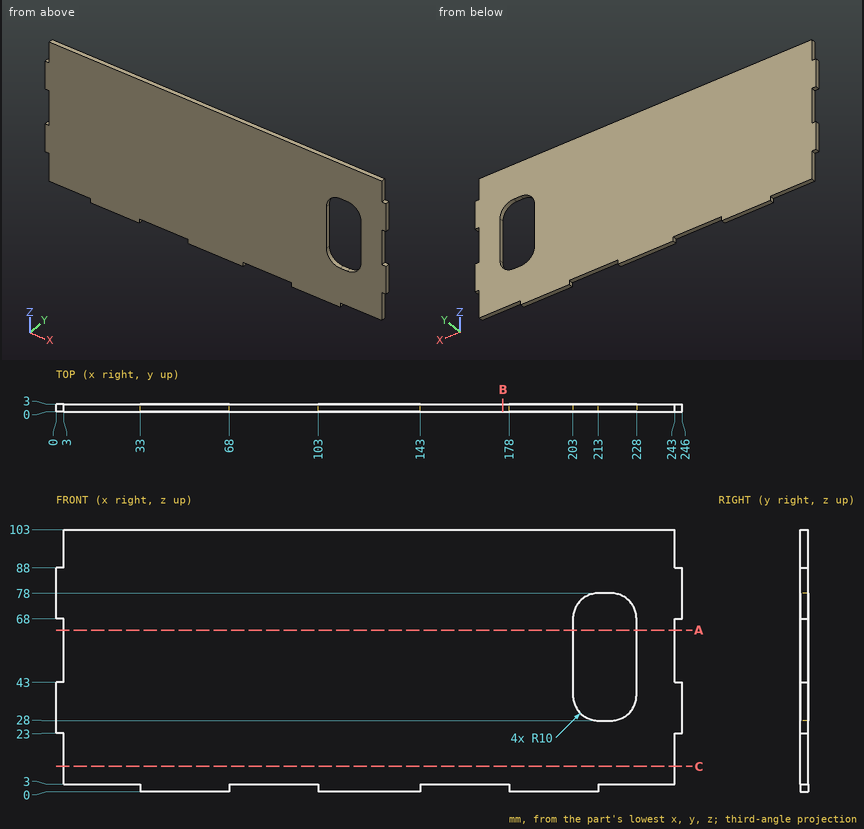
For this review, use the dimensioned drawing (mm, ordinates from the lowest corner) and the shaded views. Give positions to 0.01 mm unless a question says otherwise; leave off trailing zeros. Write each loop counter-clockwise with the first axis right and the second up, starting at its lowest first coordinate (ties: lowest second). Pieces come first, ordered by that corner, then holes. Notation, with made-up numbers: M 68,66 L 89,66 A11 cw 89,86 Z; hole C 77,71 d10. An arc over 180 degrees is marked long. Answer as a JSON object with one key per item and string values. Group by question number.
Item 1: For pin 1 Ø0.9 at (x, y) = (244.5, 2) entering from +Z; pin 2 Ø0.9 at (y, z) = (1, 1) entering from -X; pin 3 Ø1.5 at (x, y) = (17, 1.5) entering from -Z, all flat-tipped, find the tip position at first contact; note any pin that passes through.
Item 2: Consider section B-B on x = 175.5. Write out the cut boundary in (y, z).
Item 3: Consider section A-A on z = 63.5. Write out the cut boundary in (x, y).
Item 4: For probe 1 along Z at (x, y) = (219, 0.55); probe 2 along X at (y, z) = (2.1, 46); probe 3 along X at (y, z) = (1.15, 38.5), list the stretches that pass through material, from the lowest coordinate up. Write a range as [from, to].
Item 5: Consider section C-C on z = 10. Write out the cut boundary in (x, y).
Check result:
{
 "1": {"pin 1": "stops at z = 88", "pin 2": "stops at x = 33", "pin 3": "stops at z = 3"},
 "2": {"outline": "M 0,3 L 3,3 L 3,103 L 0,103 Z"},
 "3": {"outline": "M 3,0 L 203,0 L 203,3 L 3,3 Z; M 228,0 L 243,0 L 243,3 L 228,3 Z"},
 "4": {"probe 1": "z = [3, 28.05], [77.95, 103]", "probe 2": "x = [3, 203], [228, 243]", "probe 3": "x = [0, 203], [228, 246]"},
 "5": {"outline": "M 3,0 L 243,0 L 243,3 L 3,3 Z"}
}
